Could you check a few things on this model? Use its own coordinates, in mm. Face numbers are marked on the shaded views. A direction names the side the tool comes from. Round coordinates to 2 decimals unless told otherwise and drop trailing zeros. Order: outer loops, then holes, each group sorted by start corner. A loop starts at its lowest first (then second) coordinate and runs counter-clockwise, first axis right, second up. Notation, with made-up numbers: M -16,19.5 L 6,19.5 A19 cw 6,43.5 Z; hole C -35.75,14.25 d9. An arc over 180 degrees is marked long. Write each question's results on one line, items separated by ' | '. Start each with the question number.
1. Suppose I cut it at D-D on y = -53.5. Write out the boundary of the cut face in (x, z), and give its area (4 significant figures).
2. I'm going to push flat-ended pins straight in: pin 1 (0.6 mm diameter, centred on y = 60, z = -0.5, fed in from +X); pin 2 (0.6 mm diameter, centred on x = 21, z = -0.5, fed in from +Y); pin 3 (2 mm diameter, centred on x = -24.5, y = -28, fed in from -Z). Where does each tip first touch, or does it pass through?
3. Please list where these lines run through material, in increasing order: L1, parallel to X at y = -24, z = 3; L2, parallel to Z at x = 19, y = 4; L3, parallel to Z at x = 16, y = 60.5.
4. For the marked faces 1 and 2, which set-ups out of +Z, -Z, +X, -X, +Y, -Y let a thin tool reach every point of the face, with its end or its side?
5. Suppose I cut it at C-C on x = 12.5. Write out the boundary of the cut face in (y, z), and give its area (3 significant figures).
6. Suppose I cut it at A-A on y = 56.45. Write out the boundary of the cut face in (x, z).
7. Suppose I cut it at B-B on x = 21. Write out the boundary of the cut face in (y, z).
from build123d import *

# Parameters (mm, degrees)
EXTRUDE_1_DEPTH = 7.8
EXTRUDE_2_DEPTH = 1.2
SKETCH_15_4_R   = 7.5
EXTRUDE_3_DEPTH = 4
SKETCH_15_6_R   = 2
EXTRUDE_5_DEPTH = 2
SKETCH_19_W     = 1.732399473
SKETCH_19_H     = 16.304936216
SKETCH_19_H_2   = 7.781530809
EXTRUDE_6_DEPTH = 1
SKETCH_20_W     = 5.132835337
SKETCH_20_H     = 16.681714846
EXTRUDE_8_DEPTH = 1


with BuildPart() as part:
    # 草图1 → 凸台-拉伸1 (new body)
    with BuildSketch(Plane.XY):
        with BuildLine():
            Line((-26.75, -80.45), (26.75, -80.45))
            ThreePointArc((26.75, -80.45), (35.235281374, -76.935281374), (38.75, -68.45))
            Line((38.75, -68.45), (38.75, 68.45))
            ThreePointArc((38.75, 68.45), (35.235281374, 76.935281374), (26.75, 80.45))
            Line((26.75, 80.45), (-26.75, 80.45))
            ThreePointArc((-26.75, 80.45), (-35.235281374, 76.935281374), (-38.75, 68.45))
            Line((-38.75, 68.45), (-38.75, -68.45))
            ThreePointArc((-38.75, -68.45), (-35.235281374, -76.935281374), (-26.75, -80.45))
        make_face()
    extrude(amount=EXTRUDE_1_DEPTH)

    # 草图15 → 凸台-拉伸2 (add)
    with BuildSketch(Plane(origin=(0, 0, 0), x_dir=(-1, 0, 0), z_dir=(0, 0, -1))):
        with BuildLine():
            Line((-27.75, 37.45), (-5.75, 37.45))
            ThreePointArc((-5.75, 37.45), (-0.093145751, 39.793145751), (2.25, 45.45))
            Line((2.25, 45.45), (2.25, 67.45))
            ThreePointArc((2.25, 67.45), (-0.093145751, 73.106854249), (-5.75, 75.45))
            Line((-5.75, 75.45), (-27.75, 75.45))
            ThreePointArc((-27.75, 75.45), (-33.406854249, 73.106854249), (-35.75, 67.45))
            Line((-35.75, 67.45), (-35.75, 45.45))
            ThreePointArc((-35.75, 45.45), (-33.406854249, 39.793145751), (-27.75, 37.45))
        make_face()
    extrude(amount=EXTRUDE_2_DEPTH)

    # 草图15<4> → 凸台-拉伸3 (add)
    with BuildSketch(Plane(origin=(0, 0, 0), x_dir=(-1, 0, 0), z_dir=(0, 0, -1))):
        with Locations((-24.544228634, 65.45)):
            Circle(SKETCH_15_4_R)
        with Locations((-8.955771366, 56.45)):
            Circle(SKETCH_15_4_R)
        with Locations((-24.544228634, 47.45)):
            Circle(SKETCH_15_4_R)
    extrude(amount=EXTRUDE_3_DEPTH)

    # 草图15<6> → 凸台-拉伸5 (add)
    with BuildSketch(Plane(origin=(0, 0, 0), x_dir=(-1, 0, 0), z_dir=(0, 0, -1))):
        with Locations((-8.955771366, 68.45)):
            Circle(SKETCH_15_6_R)
    extrude(amount=EXTRUDE_5_DEPTH)

    # 草图19 → 凸台-拉伸6 (add)
    with BuildSketch(Plane(origin=(38.75, 0, 0), x_dir=(0, 0, -1), z_dir=(1, 0, 0))):
        with Locations((-3.974017222, 54.496659623)):
            Rectangle(SKETCH_19_W, SKETCH_19_H)
        with Locations((-3.974017222, 37.905227845)):
            Rectangle(SKETCH_19_W, SKETCH_19_H_2)
    extrude(amount=EXTRUDE_6_DEPTH)

    # 草图20 → 凸台-拉伸8 (add)
    with BuildSketch(Plane(origin=(38.75, 0, 0), x_dir=(0, 0, -1), z_dir=(1, 0, 0))):
        with Locations((-4.262343754, -17.460613504)):
            Rectangle(SKETCH_20_W, SKETCH_20_H)
    extrude(amount=-EXTRUDE_8_DEPTH)


solid = part.part
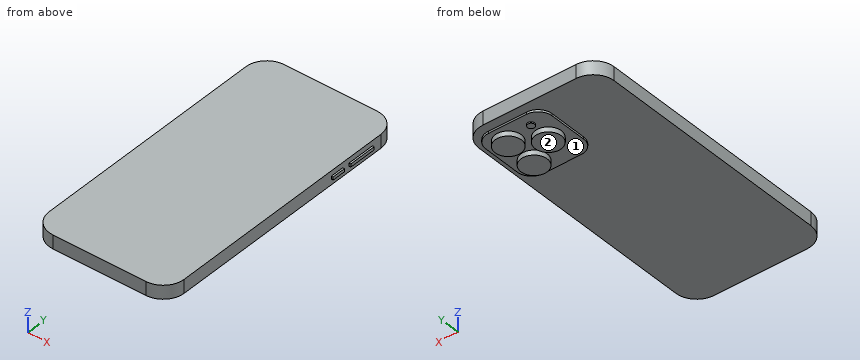
Filled sheet:
1) outline: M -38.75,0 L 38.75,0 L 38.75,7.8 L -38.75,7.8 Z | area: 604.5 mm^2
2) pin 1: stops at x = 35.75 | pin 2: stops at y = 75.45 | pin 3: stops at z = 0
3) L1: x = -38.75 to 38.75 | L2: z = 0 to 7.8 | L3: z = -1.2 to 7.8
4) face 1: -Z | face 2: -Z, +X, -X, +Y, -Y
5) outline: M -80.45,0 L 37.45,0 L 37.45,-1.2 L 49.84,-1.2 L 49.84,-4 L 63.06,-4 L 63.06,-1.2 L 75.45,-1.2 L 75.45,0 L 80.45,0 L 80.45,7.8 L -80.45,7.8 Z | area: 1,340 mm^2
6) outline: M -38.75,0 L -2.25,0 L -2.25,-1.2 L 1.46,-1.2 L 1.46,-4 L 16.46,-4 L 16.46,-1.2 L 35.75,-1.2 L 35.75,0 L 38.75,0 L 38.75,3.11 L 39.75,3.11 L 39.75,4.84 L 38.75,4.84 L 38.75,7.8 L -38.75,7.8 Z
7) outline: M -80.45,0 L 37.45,0 L 37.45,-1.2 L 40.84,-1.2 L 40.84,-4 L 54.06,-4 L 54.06,-1.2 L 58.84,-1.2 L 58.84,-4 L 72.06,-4 L 72.06,-1.2 L 75.45,-1.2 L 75.45,0 L 80.45,0 L 80.45,7.8 L -80.45,7.8 Z
